from build123d import *

# Parameters (mm, degrees)
F1_DEPTH = 3
F2_R     = 2.99999


# Not quite as in the source:
# - a fillet or chamfer is up to 0.001 mm smaller than in the source, because OpenCascade refuses the exact size


with BuildPart() as f1:
    # F0 (on Front) → F1 (new body)
    with BuildSketch(Plane.XZ):
        Polygon((0, 17.3205080757), (-10, 0), (-2.15, 0), (-2.15, 4), (2.15, 4), (2.15, 0), (10, 0), align=None)
    extrude(amount=F1_DEPTH)

    # F2 (radius 3 in the source; OpenCascade refuses exactly that, so slightly less here)
    f2_edges = [f1.edges().sort_by_distance(p)[0] for p in [
        (-5, -3, 8.660254),
        (5, -3, 8.660254),
    ]]
    fillet(f2_edges, radius=F2_R)


solid = f1.part
The listing builds one solid part. Answer for the finished solid, in the listing's coordinates (mm). A direction names the side the tool comes from. Coordinates: 2 decimals unless noted, no trailing zeros. Order: outer loops, then holes, each group sorted by start corner. A loop starts at its lowest first (then second) coordinate and runs counter-clockwise, first axis right, second up. Notation, with made-up numbers: (-38, 7.5) -> (-9, 7.5) arc R35 ccw to (-9, 41.5) -> close; hole circle Ø1 at (50.25, -9). An arc over 180 degrees is marked (long way). Answer in a Markdown table with one row per item. Add a question column.
Item 1: Which of the six approach directions +Z, -Z, +X, -X, +Y, -Y give full straight-line access (tool end or side, diameter ignored) to faces 1 (the face through (0, -1, 4)), 2 (the face through (-0.1, -3, 4.5))?
Item 2: Determine the mould class of faces 3 (the face through (-4.33, -2.1, 8.11)), 4 (the face through (-2.15, -1, 2)), 5 (the face through (-6, -1, 0)) for opening direction X: +X half, -X half, draft (parallel to the pull), parting line (faces both ways), or undercut.
Item 3: Find section A-A (y = -0.95). Write down the section's boundary in (x, z).
Item 4: Each of these flat-tipped pins is pushed along its axis until it touches: P1, Ø1.5, axis at x = -4.5, y = -0.5, coming from the +Z side; P2, Ø8, axis at x = -6.5, z = 12, coming from the -Y side; P3, Ø0.9, axis at y = -1.5, z = 3, coming from the +X side. Where does it stop, or does it pass through?
Item 5: Find the intervals of material crossed by L1, parallel to Y at x = -8, z = 2.75; L2, parallel to Z at x = 8.75, y = -0.6; L3, parallel to X at y = -2, z = 13, in increasing order. Write a range as from..to.
Result set:
| question | item | result |
|---|---|---|
| 1 | face 1 | -Z, +Y, -Y |
| 1 | face 2 | +Z, -Z, +X, -X, -Y |
| 2 | face 3 | -X half |
| 2 | face 4 | undercut |
| 2 | face 5 | draft |
| 3 | outline | (-9.82, 0) -> (-2.15, 0) -> (-2.15, 4) -> (2.15, 4) -> (2.15, 0) -> (9.82, 0) -> (0, 17.01) -> close |
| 4 | P1 | stops at z = 10.76 |
| 4 | P2 | stops at y = -2.26 |
| 4 | P3 | stops at x = 8.17 |
| 5 | L1 | y = -1.42..0 |
| 5 | L2 | z = 0..2.04 |
| 5 | L3 | x = -1.61..1.61 |
